Autodesk Inventor part; units mm, degrees
ref_plane "YZ Plane" through (0, 0, 0) normal (1, 0, 0) x (0, 1, 0)
ref_plane "XZ Plane" through (0, 0, 0) normal (0, 1, 0) x (-1, 0, 0)
ref_plane "XY Plane" through (0, 0, 0) normal (0, 0, 1) x (1, 0, 0)
sketch "Sketch1" plane through (0, 0, 0) normal (0, 0, 1) x (1, 0, 0)
  line L0 (0, 0) -> (478, 0)
  line L1 (478, 0) -> (478, 168)
  line L2 (478, 168) -> (0, 168)
  line L3 (0, 168) -> (0, 0)
  dimension "d0" = 478
  dimension "d1" = 168
extrude "Extrusion1" add sketch "Sketch1" along normal blind 10
sketch "Sketch2" plane through (0, 0, 10) normal (0, 0, 1) x (1, 0, 0)
  circle A0 centre (27.5, 134) radius 2.5
  circle A1 centre (92.5, 134) radius 2.5
  line L0 (478, 168) -> (0, 168)
  line L1 (0, 168) -> (0, 0)
  circle A2 centre (385.5, 134) radius 2.5
  circle A3 centre (450.5, 134) radius 2.5
  line L2 (478, 0) -> (478, 168)
  line L3 (27.5, 134) -> (92.5, 134) construction
  line L4 (385.5, 134) -> (450.5, 134) construction
  circle A4 centre (60, 134) radius 2.5
  circle A5 centre (418, 134) radius 2.5
  dimension "d5" = 5
  dimension "d6" = 5
  dimension "d7" = 65
  dimension "d8" = 34
  dimension "d9" = 27.5
  dimension "d10" = 5
  dimension "d11" = 5
  dimension "d12" = 65
  dimension "d13" = 27.5
  dimension "d28" = 5
  dimension "d29" = 5
extrude "Extrusion2" cut sketch "Sketch2" against normal through all
sketch "Sketch3" plane through (0, 0, 10) normal (0, 0, 1) x (1, 0, 0)
  line L0 (189, 85) -> (289, 85)
  line L1 (289, 85) -> (289, 15)
  line L2 (289, 15) -> (189, 15)
  line L3 (189, 15) -> (189, 85)
  line L4 (0, 0) -> (478, 0)
  point P0 (239, 15)
  point P1 (239, 0)
  dimension "d16" = 100
  dimension "d17" = 70
  dimension "d18" = 15
extrude "Extrusion3" [suppressed]
sketch "Sketch6" plane through (289, 15, 10) normal (-1, 0, 0) x (0, 0, 1)
  line L0 (0, 70) -> (0, 0)
  line L1 (0, 70) -> (-7, 70)
  line L2 (-7, 70) -> (-7, 0) construction
  line L3 (0, 0) -> (-7, 0)
  line L4 (-7, 70) -> (8, 70) construction
  line L5 (8, 70) -> (8, 25) construction
  line L6 (8, 25) -> (-7, 25) construction
  line L7 (-7, 25) -> (-7, 70)
  line L8 (8, 25) -> (18, 25)
  line L9 (0, -15) -> (0, 153)
  arc A0 (18, 25) -> (0, 100) centre (-131.9551, 28.6708) ccw
  line L10 (0, 100) -> (0, 70)
  line L11 (0, 70) -> (8, 70)
  line L12 (8, 70) -> (8, 25)
  point P0 (-10, -15)
  dimension "d33" = 15
  dimension "d34" = 25
  dimension "d35" = 10
  dimension "d36" = 150
  dimension "d37" = 30
extrude "Extrusion6" [suppressed]
sketch "Sketch7" plane through (189, 15, 10) normal (-1, 0, 0) x (0, 0, 1)
  arc A0 (18, 25) -> (0, 100) centre (-131.9551, 28.6708) ccw
  line L0 (18, 25) -> (0, 25)
  line L1 (0, 153) -> (0, -15)
  line L2 (0, 25) -> (0, 100)
  point P0 (-10, -15)
extrude "Extrusion7" [suppressed]
sketch "Sketch8" plane through (289, 15, 10) normal (1, 0, 0) x (0, 0, -1)
  arc A0 (0, 100) -> (-18, 25) centre (131.9551, 28.6708) ccw
  line L0 (0, 25) -> (0, 100)
  line L1 (0, 25) -> (-18, 25)
  point P0 (10, -15)
extrude "Extrusion8" [suppressed]
sketch "Sketch9" plane through (0, 0, 10) normal (0, 0, 1) x (1, 0, 0)
  line L0 (214, 25) -> (264, 25) construction
  circle A0 centre (264, 25) radius 12.5
  circle A1 centre (214, 25) radius 12.5
  line L1 (0, 0) -> (478, 0) construction
  point P0 (239, 25)
  point P1 (239, 0)
  dimension "d45" = 50
  dimension "d46" = 25
  dimension "d47" = 25
  dimension "d48" = 25
extrude "Extrusion9" cut sketch "Sketch9" against normal through all
properties part number "TC005b" material "ABS Plastic"
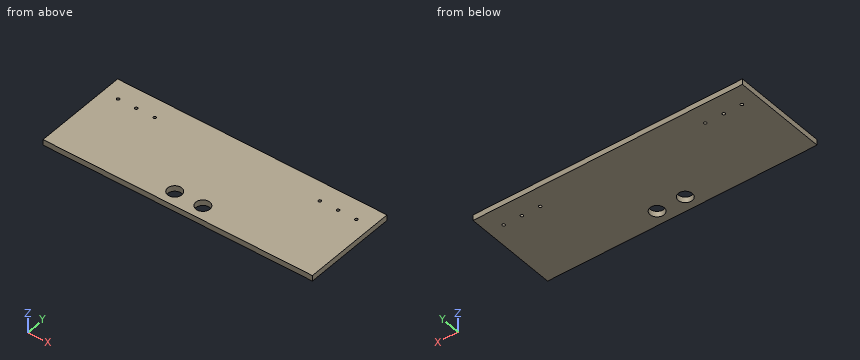
The model under review builds one solid part; all positions refer to its coordinate system, in mm. Give positions to 0.01 mm unless a question says otherwise; leave off trailing zeros. Order: outer loops, then holes, each group sorted by start corner. A loop starts at its lowest first (then second) coordinate and runs counter-clockwise, first axis right, second up. Notation, with made-up numbers: (11.5, 33) - (53.5, 33) arc R19 ccw to (53.5, 56) - close; hole circle Ø11 at (22.5, 64.25). An arc over 180 degrees is marked (long way). Use CSV: the item, a comma, the result in double quotes. Start each with the question number.
Q1. Clearance check with flat-ended pins moving along their axes: pin 1 Ø3 at (x, y) = (385.5, 134) entering from +Z; pin 2 Ø1.5 at (x, y) = (245.5, 34.5) entering from -Z. State where each tip first meets the part, or that it passes through.
Q2. To check wall thickness, follow line 1 along Y through (x, z) = (214, 2.75); line 2 along X through (y, z) = (23, 5); line 3 along X through (y, z) = (27.5, 4.25). State the ranges of each line that lie inside material, in increasing order. Write a range as [from, to].
Q3. We need section A-A, the plane x = 214. Write out the cut boundary in (y, z), and give its area (3 significant figures).
Outcome:
1,pin 1,"passes through"
1,pin 2,"stops at z = 0"
2,line 1,"y = [0, 12.5], [37.5, 168]"
2,line 2,"x = [0, 201.66], [226.34, 251.66], [276.34, 478]"
2,line 3,"x = [0, 201.75], [226.25, 251.75], [276.25, 478]"
3,outline,"(0, 0) - (12.5, 0) - (12.5, 10) - (0, 10) - close; (37.5, 0) - (168, 0) - (168, 10) - (37.5, 10) - close"
3,area,"1,430 mm^2"
